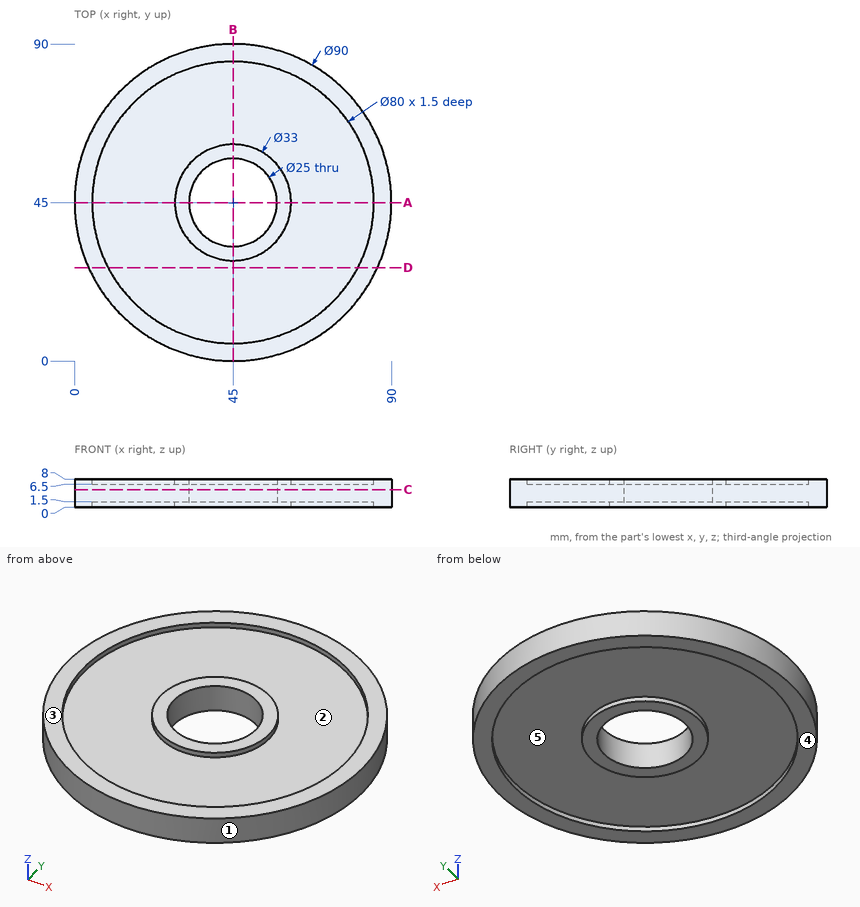
Study the drawing (mm; zero at the part's minimum x, y, z) and answer. A direction names the side the tool comes from. Round coordinates to 2 decimals unless told otherwise and drop trailing zeros. Loops run counter-clockwise (first coordinate to the right, second up) from the corner with the lowest first, then second, coordinate; pieces in that order, holes last.
Q1. Which of the six approach directions +Z, -Z, +X, -X, +Y, -Y give full straight-line access (tool end or side, diameter ignored) to the marked faces 4 and 5?
Q2. For a pull along X with two mould halves and no side action, classify the marked faces 1, 2 and 3 as released by +X, released by -X, zero draft, split by the parting line, or undercut.
Q3. Section A-A, the plane y = 45 is taken. Determine the outline of the cut face in (x, z), then the cut area to 3 significant figures.
Q4. Given pin 1 Ø8 at (x, y) = (62.5, 69) entering from -Z; pin 2 Ø10 at (x, y) = (74.5, 55.5) entering from +Z; pin 3 Ø1.5 at (y, z) = (47, 1) entering from +X; pin 4 Ø22.5 at (x, y) = (45, 45) entering from -Z, each flat-ended and moving along its own axis, determine where each tip first touches the part or whether it passes through.
Q5. Section C-C, the plane z = 5 is taken. Determine the outline of the cut face in (x, y).
Q6. Find the intervals of material crossed by line 1 (X direction, y = 45, z = 6.85); line 2 (X direction, y = 45, z = 5), in increasing order.
Q7. Section D-D, the plane y = 26.5 is taken. Determine the outline of the cut face in (x, z), then the cut area to 3 significant figures.
Completed:
1. face 4: -Z, +X, -X, +Y, -Y
1. face 5: -Z
2. face 1: split by the parting line
2. face 2: undercut
2. face 3: zero draft
3. outline: (0, 0) - (5, 0) - (5, 1.5) - (28.5, 1.5) - (28.5, 0) - (32.5, 0) - (32.5, 8) - (28.5, 8) - (28.5, 6.5) - (5, 6.5) - (5, 8) - (0, 8) - close; (57.5, 0) - (61.5, 0) - (61.5, 1.5) - (85, 1.5) - (85, 0) - (90, 0) - (90, 8) - (85, 8) - (85, 6.5) - (61.5, 6.5) - (61.5, 8) - (57.5, 8) - close
3. area: 379 mm2
4. pin 1: stops at z = 1.5
4. pin 2: stops at z = 6.5
4. pin 3: stops at x = 89.98
4. pin 4: passes through
5. outline: circle Ø90 at (45, 45); hole circle Ø25 at (45, 45)
6. line 1: x = 0 to 5, 28.5 to 32.5, 57.5 to 61.5, 85 to 90
6. line 2: x = 0 to 32.5, 57.5 to 90
7. outline: (3.98, 0) - (9.54, 0) - (9.54, 1.5) - (80.46, 1.5) - (80.46, 0) - (86.02, 0) - (86.02, 8) - (80.46, 8) - (80.46, 6.5) - (9.54, 6.5) - (9.54, 8) - (3.98, 8) - close
7. area: 444 mm2
